Geometry: final body of the model. Coordinates: model frame, mm. A direction names the side the tool comes from. Give positions to 0.01 mm unless a question says otherwise; leave off trailing zeros. Write each loop counter-clockwise with the first axis right and the second up, starting at its lowest first coordinate (ties: lowest second). Pieces come first, ordered by that corner, then holes. Notation, with made-up numbers: (82.5, 32.5) -> (126.5, 32.5) arc R28 ccw to (126.5, 52.5) -> close; hole circle Ø4 at (20, 35.5). An arc over 180 degrees is marked (long way). Answer in a Markdown table with one row per item. Add a question column.
from build123d import *

# Parameters (mm, degrees)
F1_DEPTH = 26.416
F2_W     = 96.342794
F2_H     = 45.070231
F3_DEPTH = 22.098


with BuildPart() as f1:
    # F0 (on Front) → F1 (new body)
    with BuildSketch(Plane.XZ):
        with BuildLine():
            Line((42.877077, 52.316071), (-42.193984, 52.316071))
            ThreePointArc((-42.193984, 52.316071), (-50.806357, 48.748709), (-54.373719, 40.136336))
            Line((-54.373719, 40.136336), (-54.373719, 4.850378))
            ThreePointArc((-54.373719, 4.850378), (-50.957663, -3.396709), (-42.710576, -6.812765))
            Line((-42.710576, -6.812765), (-25.95896, -6.812765))
            Line((-25.95896, -6.812765), (23.615748, -6.812765))
            Line((23.615748, -6.812765), (44.507051, -6.812765))
            ThreePointArc((44.507051, -6.812765), (51.483839, -3.922885), (54.373719, 3.053903))
            Line((54.373719, 3.053903), (54.373719, 40.81943))
            ThreePointArc((54.373719, 40.81943), (51.006431, 48.948783), (42.877077, 52.316071))
        make_face()
        with BuildLine():
            ThreePointArc((-48.378143, 43.012887), (-47.65402, 44.761075), (-45.905832, 45.485198))
            Line((-45.905832, 45.485198), (42.722448, 45.485198))
            ThreePointArc((42.722448, 45.485198), (46.721629, 43.828684), (48.378143, 39.829503))
            Line((48.378143, 39.829503), (48.378143, 3.861538))
            ThreePointArc((48.378143, 3.861538), (47.252429, 1.143823), (44.534713, 0.018108))
            Line((44.534713, 0.018108), (-45.961362, 0.018108))
            ThreePointArc((-45.961362, 0.018108), (-47.670285, 0.725967), (-48.378143, 2.434889))
            Line((-48.378143, 2.434889), (-48.378143, 43.012887))
        make_face(mode=Mode.SUBTRACT)
        Polygon((23.615748, -6.812765), (-25.95896, -6.812765), (-40.935349, -28.11721), (43.002788, -28.11721), align=None)
    extrude(amount=F1_DEPTH)

    # F2 (on Front) → F3 (join)
    with BuildSketch(Plane.XZ):
        with Locations((0, 22.535115)):
            Rectangle(F2_W, F2_H)
    extrude(amount=F3_DEPTH)


solid = f1.part
Q1. Section B-B on z = 7.5. Return loops of the section in (x, y).
Q2. Access query for faces 5 (the flat face through (-33.342, -13.023, -17.316)), 6 (the flat face through (0, -24, 0.018)), 7 (the flat face through (48.171, -11, 22)). Directions: +Z, -Z, +X, -X, +Y, -Y. A direction counts if a zero-diameter tool reaches every point of the face in a straight line with its end or side. Return the directions, or none.
Q3. Line query: probe 1 along X at (y, z) = (-12.25, 18); probe 2 along Z at (x, y) = (-15, -10.25); probe 3 along Z at (x, y) = (8.5, -25). Output: solid intervals per line, ascending. Write a range as from..to.
Q4. Section A-A on y = -17. Return loops of the section in (x, z), and give its area (3 significant figures).
Q5. Section C-C on x = -29. Return loops of the section in (y, z).
Q6. Contact query for flat-ended pins moving along their axis: pin 1 Ø1.5 at (y, z) = (-7, -13.5) entering from -X; pin 2 Ø4 at (x, z) = (11.5, 11.5) entering from +Y; pin 3 Ø13.5 at (x, z) = (0.5, 26) entering from -Y. Output: stop coordinate, or through.
Q7. Section D-D on x = -16. Return loops of the section in (y, z).
Q8. Pull-direction query (X, two-part tool) for faces 1 (the flat face through (-54.374, -13, 23)), 2 (the flat face through (48.378, -13, 22)), 3 (the flat face through (-48.171, -11, 22)), 4 (the flat face through (-1, 0, 13)); classes: +X half, -X half, draft (parallel to the pull), parting line (faces both ways), or undercut.
Checks:
| question | item | result |
|---|---|---|
| 1 | outline | (-54.37, -26.42) -> (-48.38, -26.42) -> (-48.38, 0) -> (-54.37, 0) -> close; (-48.17, -22.1) -> (48.17, -22.1) -> (48.17, 0) -> (-48.17, 0) -> close; (48.38, -26.42) -> (54.37, -26.42) -> (54.37, 0) -> (48.38, 0) -> close |
| 2 | face 5 | -X, +Y, -Y |
| 2 | face 6 | -Y |
| 2 | face 7 | +Y, -Y |
| 3 | probe 1 | -54.37..-48.38, -48.17..48.17, 48.38..54.37 |
| 3 | probe 2 | -28.12..45.07, 45.49..52.32 |
| 3 | probe 3 | -28.12..0.02, 45.49..52.32 |
| 4 | outline | (-54.37, 4.85) arc R11.66 ccw to (-42.71, -6.81) -> (-25.96, -6.81) -> (-40.94, -28.12) -> (43, -28.12) -> (23.62, -6.81) -> (44.51, -6.81) arc R9.87 ccw to (54.37, 3.05) -> (54.37, 40.82) arc R11.5 ccw to (42.88, 52.32) -> (-42.19, 52.32) arc R12.18 ccw to (-54.37, 40.14) -> close; hole (-48.38, 2.43) arc R2.42 ccw to (-48.17, 1.46) -> (-48.17, 44) arc R2.47 ccw to (-48.38, 43.01) -> close; hole (-47.28, 45.07) -> (44.85, 45.07) arc R5.66 ccw to (42.72, 45.49) -> (-45.91, 45.49) arc R2.47 ccw to start; hole (48.17, 2.62) arc R3.84 ccw to (48.38, 3.86) -> (48.38, 39.83) arc R5.66 ccw to (48.17, 41.34) -> close |
| 4 | area | 7,690 mm^2 |
| 5 | outline | (-26.42, -28.12) -> (0, -28.12) -> (0, -11.14) -> (-26.42, -11.14) -> close; (-26.42, -6.81) -> (0, -6.81) -> (0, 45.07) -> (-22.1, 45.07) -> (-22.1, 0.02) -> (-26.42, 0.02) -> close; (-26.42, 45.49) -> (0, 45.49) -> (0, 52.32) -> (-26.42, 52.32) -> close |
| 6 | pin 1 | x = -31.19 |
| 6 | pin 2 | y = 0 |
| 6 | pin 3 | y = -22.1 |
| 7 | outline | (-26.42, -28.12) -> (0, -28.12) -> (0, 45.07) -> (-22.1, 45.07) -> (-22.1, 0.02) -> (-26.42, 0.02) -> close; (-26.42, 45.49) -> (0, 45.49) -> (0, 52.32) -> (-26.42, 52.32) -> close |
| 8 | face 1 | -X half |
| 8 | face 2 | undercut |
| 8 | face 3 | undercut |
| 8 | face 4 | draft |
